Could you check a few things on this model? Use its own coordinates, in mm. Face numbers are marked on the shaded views. Coordinates: 2 decimals unless noted, no trailing zeros. Order: outer loops, then holes, each group sorted by start corner. A loop starts at its lowest first (then second) coordinate and runs counter-clockwise, first axis right, second up. Notation, with made-up numbers: (27.25, 76.5) -> (34.25, 76.5) arc R21 ccw to (34.25, 114.5) -> close; hole circle Ø2 at (-13, 16.25). An arc over 180 degrees is marked (long way). Return JSON: item names as keys, results as strings. Group by question number.
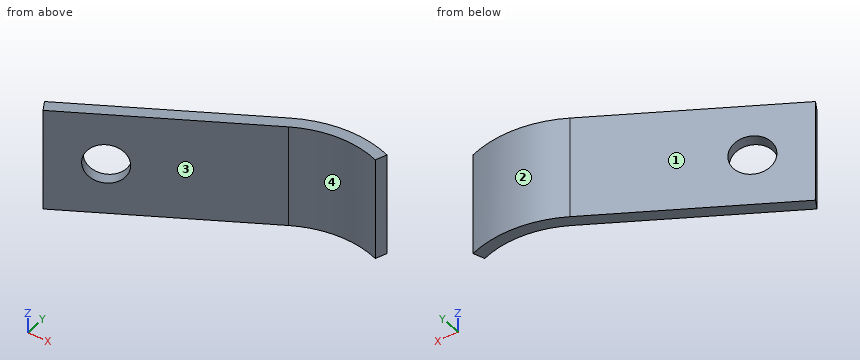
from build123d import *

# Parameters (mm, degrees)
EXTRUDE_1_DEPTH     = 9
SKETCH_2_R          = 3.5
CUT_EXTRUDE_1_DEPTH = 18


with BuildPart() as part:
    # 草图1 → 凸台-拉伸1 (new, symmetric)
    with BuildSketch(Plane.XY):
        with BuildLine():
            Line((-38.810889132, -2.777568136), (-8.5, 14.722431864))
            ThreePointArc((-8.5, 14.722431864), (-1.481647627, 16.935309868), (5.814342437, 15.974774553))
            Line((5.814342437, 15.974774553), (6.498382723, 17.854159795))
            ThreePointArc((6.498382723, 17.854159795), (-1.655959112, 18.927699264), (-9.5, 16.454482672))
            Line((-9.5, 16.454482672), (-39.810889132, -1.045517328))
            Line((-39.810889132, -1.045517328), (-38.810889132, -2.777568136))
        make_face()
    extrude(amount=EXTRUDE_1_DEPTH, both=True)

    # 草图2 → 切除-拉伸1 (cut)
    with BuildSketch(Plane(origin=(-9.5, 16.454482672, 0), x_dir=(0.8660254037844398, 0.49999999999999806, 0), z_dir=(-0.49999999999999806, 0.8660254037844398, 0))):
        with Locations(Location((-26, 0, 0), (0, 0, 180))):
            Circle(SKETCH_2_R)
    extrude(amount=-CUT_EXTRUDE_1_DEPTH, mode=Mode.SUBTRACT)


solid = part.part
Q1. I'm going to push flat-ended pins straight in: pin 1 Ø10 at (x, y) = (-26.5, 15.5) entering from -Z; pin 2 Ø1.5 at (y, z) = (0, 4) entering from +X; pin 3 Ø5 at (x, z) = (-0.5, 3) entering from -Y; pin 4 Ø3 at (x, z) = (-29, 2) entering from -Y. Where does each tip first touch, or does it pass through?
Q2. I want a section at A-A on z = 1. Please give me the cut outline in (x, y), and give its area (3 significant figures).
Q3. We'd pull the mould along X, two halves only. Please class the marked faces 1, 2, 3 and 4: pulls with the +X half, pulls with the -X half, needs draft (parallel to the pull), parting line crosses it, or undercut.
Q4. I want a section at B-B on z = 7.75. Please give me the cut outline in (x, y), and give its area (3 significant figures).
Q5. I want a section at D-D on z = -2. Please give me the cut outline in (x, y).
Q6. I want a section at C-C on x = 0. Please give me the cut outline in (y, z).
Q7. I need wall thicknesses on line 1 along Z through (x, y) = (-31, 3.5); line 2 along X through (y, z) = (6.5, 0.25); line 3 along Y through (x, z) = (-34, -2.25). Which ranges of each line are inside material? Lowest first, please. Write a range as from..to.
Response values:
{
 "1": {"pin 1": "passes through", "pin 2": "stops at x = -32.7", "pin 3": "stops at y = 16.73", "pin 4": "stops at y = 2.39"},
 "2": {"outline": "(-39.81, -1.05) -> (-38.81, -2.78) -> (-33.92, 0.05) -> (-34.92, 1.78) -> close; (-29.11, 5.13) -> (-28.11, 3.4) -> (-8.5, 14.72) arc R17 cw to (5.81, 15.97) -> (6.5, 17.85) arc R19 ccw to (-9.5, 16.45) -> close", "area": "88.0 mm²"},
 "3": {"face 1": "pulls with the -X half", "face 2": "parting line crosses it", "face 3": "pulls with the +X half", "face 4": "undercut"},
 "4": {"outline": "(-39.81, -1.05) -> (-38.81, -2.78) -> (-8.5, 14.72) arc R17 cw to (5.81, 15.97) -> (6.5, 17.85) arc R19 ccw to (-9.5, 16.45) -> close", "area": "101 mm²"},
 "5": {"outline": "(-39.81, -1.05) -> (-38.81, -2.78) -> (-33.5, 0.29) -> (-34.5, 2.02) -> close; (-29.53, 4.89) -> (-28.53, 3.16) -> (-8.5, 14.72) arc R17 cw to (5.81, 15.97) -> (6.5, 17.85) arc R19 ccw to (-9.5, 16.45) -> close"},
 "6": {"outline": "(17, -9) -> (19, -9) -> (19, 9) -> (17, 9) -> close"},
 "7": {"line 1": "z = -9..-3.38, 3.38..9", "line 2": "x = -26.74..-22.74", "line 3": "y = 0..1.53"}
}
